Geometry check sheet. Reference: the model listing, model coordinates, mm. Face numbers are marked on the shaded views. Coordinates: 2 decimals unless noted, no trailing zeros. Loops run counter-clockwise (first coordinate to the right, second up) from the corner with the lowest first, then second, coordinate; pieces in that order, holes last.
from build123d import *

# Parameters (mm, degrees)
EXTRUDE1_DEPTH    = 5
SKETCH2_R         = 5
EXTRUDE2_DEPTH    = 10
SKETCH3_OUTSIDE_W = 48.43
SKETCH3_OUTSIDE_H = 51.524
SKETCH3_OUTSIDE_R = 10
EXTRUDE4_DEPTH    = 10
EXTRUDE4_TAPER    = 45
SKETCH4_OUTSIDE_W = 48.43
SKETCH4_OUTSIDE_H = 51.524
SKETCH4_OUTSIDE_R = 10
EXTRUDE5_DEPTH    = 10
EXTRUDE5_TAPER    = 45


with BuildPart() as part:
    # Sketch1 → Extrude1 (new, symmetric)
    with BuildSketch(Plane.XY):
        Polygon((0, 11.547005384), (-10, 5.773502692), (-10, -5.773502692), (0, -11.547005384), (10, -5.773502692), (10, 5.773502692), align=None)
    extrude(amount=EXTRUDE1_DEPTH, both=True)

    # Sketch2 → Extrude2 (cut)
    with BuildSketch(Plane.XY.offset(5)):
        Circle(SKETCH2_R)
    extrude(amount=-EXTRUDE2_DEPTH, mode=Mode.SUBTRACT)

    # Sketch3 outside → Extrude4 (cut)
    with BuildSketch(Plane.XY.offset(5)):
        Rectangle(SKETCH3_OUTSIDE_W, SKETCH3_OUTSIDE_H)
        Circle(SKETCH3_OUTSIDE_R, mode=Mode.SUBTRACT)
    extrude(amount=-EXTRUDE4_DEPTH, taper=EXTRUDE4_TAPER, mode=Mode.SUBTRACT)

    # Sketch4 outside → Extrude5 (cut)
    with BuildSketch(Plane(origin=(0, 0, -5), x_dir=(-1, 0, 0), z_dir=(0, 0, -1))):
        Rectangle(SKETCH4_OUTSIDE_W, SKETCH4_OUTSIDE_H)
        Circle(SKETCH4_OUTSIDE_R, mode=Mode.SUBTRACT)
    extrude(amount=-EXTRUDE5_DEPTH, taper=EXTRUDE5_TAPER, mode=Mode.SUBTRACT)


solid = part.part
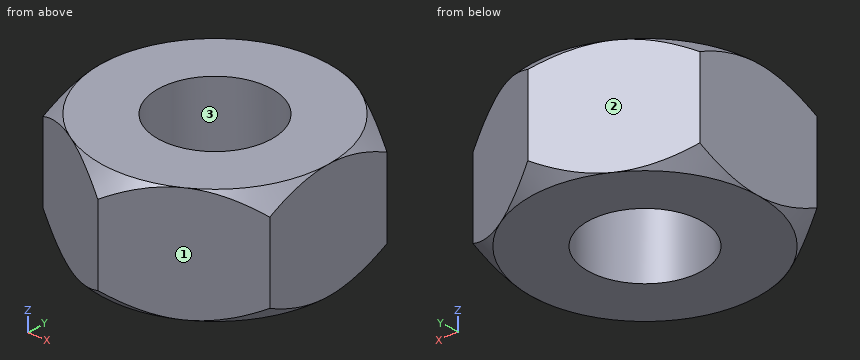
(1) Draft check along X on the marked faces 1, 2 and 3. Enter one of: +X half, -X half, draft (parallel to the pull), parting line (faces both ways), or undercut.
Findings:
face 1: +X half
face 2: -X half
face 3: undercut
(2) Gauge pin test, flat ends, axial feed: pin 1 Ø2 at (x, z) = (0.5, -2.5) entering from +Y; pin 2 Ø4 at (x, z) = (-7, 3) entering from +Y; pin 3 Ø6 at (x, z) = (-6.5, -0.5) entering from +Y. Record the tip position at first contact, or that the pin passes through.
Findings:
pin 1: stops at y = 11.55
pin 2: stops at y = 8.66
pin 3: stops at y = 9.53
(3) Sectioned sample at A-A on z = -1.25. Record the cut outline in (x, y).
Findings:
outline: (-10, -5.77) - (0, -11.55) - (10, -5.77) - (10, 5.77) - (0, 11.55) - (-10, 5.77) - close; hole circle Ø10 at (0, 0)
(4) Scan lines: L1, parallel to X at y = -2, z = 0.75; L2, parallel to Y at x = -4, z = 0; L3, parallel to X at y = -3.5, z = -0.5. Record each from-to range of solid material in increasing order.
Findings:
L1: x = -10 to -4.58, 4.58 to 10
L2: y = -9.24 to -3, 3 to 9.24
L3: x = -10 to -3.57, 3.57 to 10
